Verification items for the finished model (mm, model axes). Face numbers are marked on the shaded views. Coordinates: 2 decimals unless noted, no trailing zeros. Write each loop counter-clockwise with the first axis right and the second up, starting at its lowest first coordinate (ties: lowest second). Pieces come first, ordered by that corner, then holes. Notation, with made-up numbers: (48, -10) -> (96, -10) arc R38 ccw to (96, 29) -> close; hole circle Ø9 at (19.5, -28). An arc over 180 degrees is marked (long way). Answer in a Markdown table with one row per item.
```python
from build123d import *

# Parameters (mm, degrees)
SKETCH1_W                     = 52
SKETCH1_H                     = 16.25
CLAMP_LOWER_HALF_DEPTH        = 20
HANDLEBAR_BORE_DEPTH          = 44.783558558
HANDLEBAR_BORE_DEPTH_BACK     = 44.783558558
SKETCH2_R                     = 12.1
M5_CLEARANCE_HOLES_DEPTH      = 44.783558558
M5_CLEARANCE_HOLES_DEPTH_BACK = 44.783558558
SKETCH3_R                     = 2.75


with BuildPart() as part:
    # Sketch1 → Clamp Lower Half (new, symmetric)
    with BuildSketch(Plane(origin=(0, 0, 0), x_dir=(0, 0, -1), z_dir=(1, 0, 0))):
        with Locations((0, -20.875)):
            Rectangle(SKETCH1_W, SKETCH1_H)
    extrude(amount=CLAMP_LOWER_HALF_DEPTH, both=True)

    # Sketch2 → Handlebar Bore (cut, two sides: drawn at the far end of the back side and taken through both)
    with BuildSketch(Plane(origin=(0, 0, 0), x_dir=(0, 0, -1), z_dir=(1, 0, 0)).offset(-HANDLEBAR_BORE_DEPTH_BACK)):
        with Locations((0, -12)):
            Circle(SKETCH2_R)
    extrude(amount=HANDLEBAR_BORE_DEPTH + HANDLEBAR_BORE_DEPTH_BACK, mode=Mode.SUBTRACT)

    # Sketch3 → M5 Clearance Holes (cut, two sides: drawn at the far end of the back side and taken through both)
    with BuildSketch(Plane(origin=(0, 0, 0), x_dir=(1, 0, 0), z_dir=(0, 1, 0)).offset(-M5_CLEARANCE_HOLES_DEPTH_BACK)):
        with Locations(Location((0, -18.5, 0), (0, 0, 270))):
            Circle(SKETCH3_R)
        with Locations(Location((0, 18.5, 0), (0, 0, 270))):
            Circle(SKETCH3_R)
    extrude(amount=M5_CLEARANCE_HOLES_DEPTH + M5_CLEARANCE_HOLES_DEPTH_BACK, mode=Mode.SUBTRACT)


solid = part.part
```
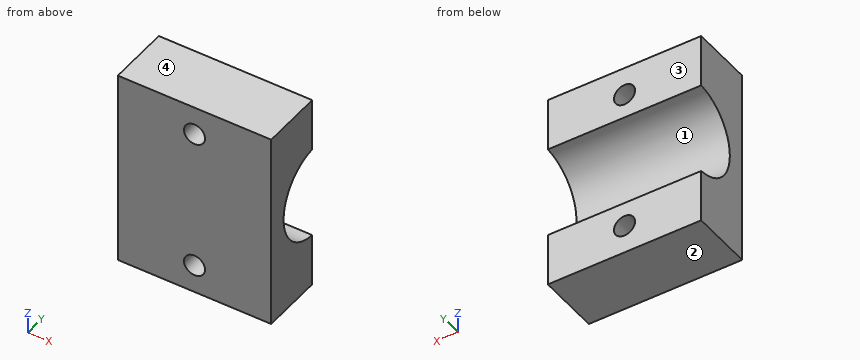
1. Sectioned sample at B-B, the plane z = 18.5. Record the cut outline in (x, y), and give its area (3 significant figures).
Findings below:
| item | result |
|---|---|
| outline | (-20, -29) -> (-2.75, -29) -> (-2.75, -12.75) -> (-20, -12.75) -> close; (2.75, -29) -> (20, -29) -> (20, -12.75) -> (2.75, -12.75) -> close |
| area | 561 mm² |
2. Release check for a two-part mould opening along Z. For the marked faces 1, 2, 3 and 4 record: released by +Z, released by -Z, zero draft, split by the parting line, or undercut.
Findings below:
| item | result |
|---|---|
| face 1 | undercut |
| face 2 | released by -Z |
| face 3 | zero draft |
| face 4 | released by +Z |
3. Sectioned sample at A-A, the plane x = 0. Record the cut outline in (y, z).
Findings below:
| item | result |
|---|---|
| outline | (-29, -26) -> (-12.75, -26) -> (-12.75, -21.25) -> (-29, -21.25) -> close; (-29, -15.75) -> (-12.75, -15.75) -> (-12.75, -12.08) arc R12.1 cw to (-12.75, 12.08) -> (-12.75, 15.75) -> (-29, 15.75) -> close; (-29, 21.25) -> (-12.75, 21.25) -> (-12.75, 26) -> (-29, 26) -> close |
4. Material ranges on probe 1 along Z at (x, y) = (0, -20.5); probe 2 along Z at (x, y) = (0, -21); probe 3 along X at (y, z) = (-18.25, -18.5), recorded low to high. Write a range as from..to.
Findings below:
| item | result |
|---|---|
| probe 1 | z = -26..-21.25, -15.75..-8.61, 8.61..15.75, 21.25..26 |
| probe 2 | z = -26..-21.25, -15.75..-8.09, 8.09..15.75, 21.25..26 |
| probe 3 | x = -20..-2.75, 2.75..20 |
5. Sectioned sample at D-D, the plane x = 11. Record the cut outline in (y, z), and give its area (3 significant figures).
Findings below:
| item | result |
|---|---|
| outline | (-29, -26) -> (-12.75, -26) -> (-12.75, -12.08) arc R12.1 cw to (-12.75, 12.08) -> (-12.75, 26) -> (-29, 26) -> close |
| area | 633 mm² |
6. Sectioned sample at C-C, the plane y = -17. Record the cut outline in (x, z).
Findings below:
| item | result |
|---|---|
| outline | (-20, -26) -> (20, -26) -> (20, -11.02) -> (-20, -11.02) -> close; (-20, 11.02) -> (20, 11.02) -> (20, 26) -> (-20, 26) -> close; hole circle Ø5.5 at (0, -18.5); hole circle Ø5.5 at (0, 18.5) |
7. Go/stop test with flat-tipped pins: pin 1 (3.5 mm diameter, centred on x = 0, z = 18.5, fed in from +Y); pin 2 (1.5 mm diameter, centred on x = -3.5, z = 1, fed in from +Y); pin 3 (1 mm diameter, centred on x = 8.5, z = 9.5, fed in from +Y). Record where each tip stops, or that it passes through.
Findings below:
| item | result |
|---|---|
| pin 1 | passes through |
| pin 2 | stops at y = -23.97 |
| pin 3 | stops at y = -18.81 |
